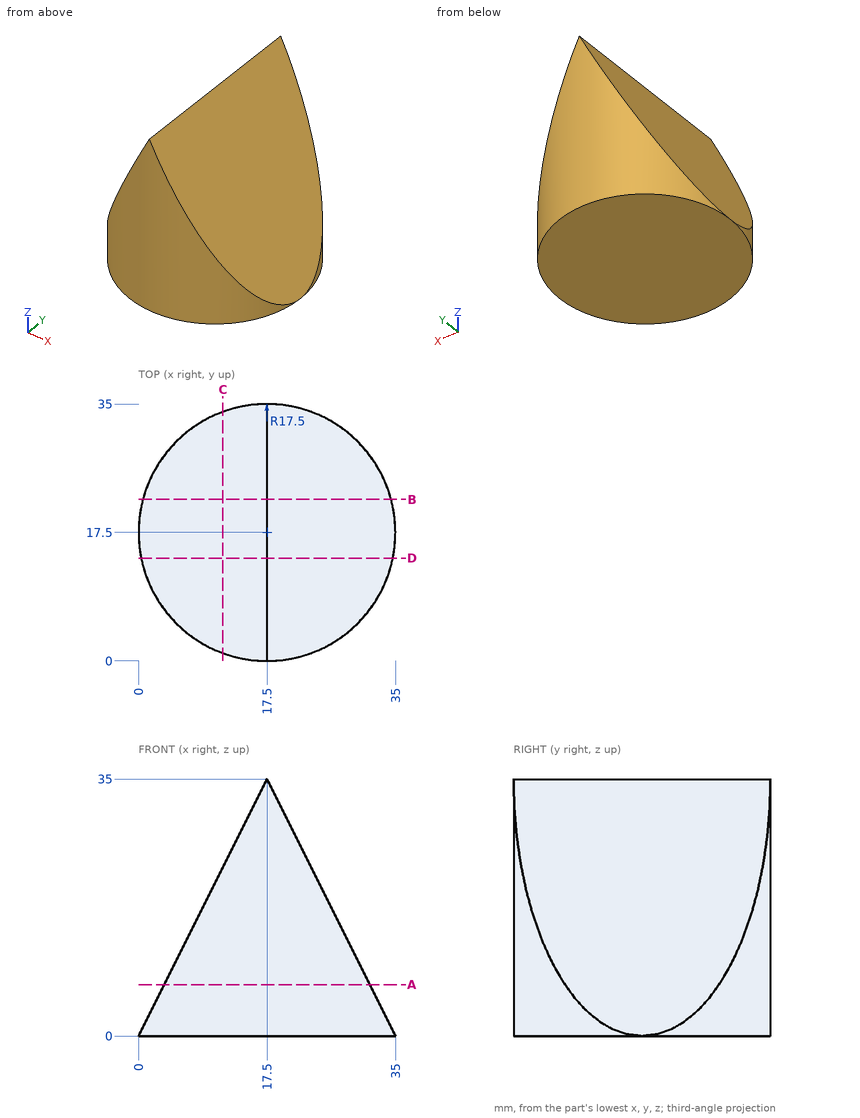
Job drawing, mm, ordinate dimensions from the low corner. One solid piece. Coordinates: 2 decimals unless noted, no trailing zeros. Write each loop counter-clockwise with the first axis right and the second up, starting at its lowest first coordinate (ties: lowest second). Pieces come first, ordered by that corner, then holes. Notation, with made-up numbers: M 57,52 L 77,52 A26 cw 77,71 Z; hole C -2,77 d10. An arc over 180 degrees is marked long. Answer as a JSON object with one key per item and string values. Group by question number.
1) Saw through at A-A (z = 7). Write the cut outline in (x, y).
2) Saw through at B-B (y = 22). Write the cut outline in (x, z).
3) Saw through at C-C (x = 11.5). Write the cut outline in (y, z).
4) Pin check, flat tips, straight feed: pin 1 Ø8 at (x, y) = (15, 15) entering from +Z; pin 2 Ø8 at (x, z) = (8.5, 10.5) entering from +Y; pin 3 Ø12 at (x, y) = (24.5, 11.5) entering from +Z. Stop position of each tip, or through.
5) Wall check: line 1 (Y direction, x = 23, z = 14); line 2 (Z direction, x = 7.5, y = 28); line 3 (X direction, y = 27, z = 20.5). Give the ranges that are in metal, low to high. Write a range as from..to.
6) Saw through at D-D (y = 14). Write the cut outline in (x, z).
Values follow:
{
 "1": {"outline": "M 3.5,7 A17.5 ccw 31.5,7 L 31.5,28 A17.5 ccw 3.5,28 Z"},
 "2": {"outline": "M 0.59,0 L 34.41,0 L 34.41,1.18 L 17.5,35 L 0.59,1.18 Z"},
 "3": {"outline": "M 1.06,0 L 33.94,0 L 33.94,23 L 1.06,23 Z"},
 "4": {"pin 1": "stops at z = 35", "pin 2": "stops at y = 34.27", "pin 3": "stops at z = 33"},
 "5": {"line 1": "y = 0.89..34.11", "line 2": "z = 0..15", "line 3": "x = 10.25..24.75"},
 "6": {"outline": "M 0.35,0 L 34.65,0 L 34.65,0.71 L 17.5,35 L 0.35,0.71 Z"}
}
